from build123d import *

# Parameters (mm, degrees)
BOSS_EXTRUDE1_DEPTH      = 40
BOSS_EXTRUDE1_DEPTH_BACK = 40
SKETCH1_W                = 30
SKETCH1_H                = 40
CUT_EXTRUDE1_DEPTH       = 80
CUT_EXTRUDE1_DEPTH_BACK  = 80
SKETCH2_R                = 4.05
CUT_EXTRUDE2_START       = 15
SKETCH3_R                = 7
CUT_EXTRUDE2_DEPTH       = 6
CUT_EXTRUDE3_DEPTH       = 36
CUT_EXTRUDE3_DEPTH_BACK  = 36


with BuildPart() as part:
    # Sketch1 → Boss-Extrude1 (new, two sides: drawn at the far end of the back side and taken through both)
    with BuildSketch(Plane.XY.offset(-BOSS_EXTRUDE1_DEPTH_BACK)):
        Rectangle(SKETCH1_W, SKETCH1_H)
    extrude(amount=BOSS_EXTRUDE1_DEPTH + BOSS_EXTRUDE1_DEPTH_BACK)

    # Sketch2 → Cut-Extrude1 (cut, two sides: drawn at the far end of the back side and taken through both)
    with BuildSketch(Plane(origin=(0, 0, 0), x_dir=(0, 0, -1), z_dir=(1, 0, 0)).offset(-CUT_EXTRUDE1_DEPTH_BACK)):
        with Locations((-20, 0)):
            Circle(SKETCH2_R)
        with Locations((20, 0)):
            Circle(SKETCH2_R)
    extrude(amount=CUT_EXTRUDE1_DEPTH + CUT_EXTRUDE1_DEPTH_BACK, mode=Mode.SUBTRACT)

    # Sketch3 → Cut-Extrude2 (cut)
    with BuildSketch(Plane(origin=(0, 0, 0), x_dir=(0, 0, -1), z_dir=(1, 0, 0)).offset(CUT_EXTRUDE2_START)):
        with Locations((-20, 0)):
            Circle(SKETCH3_R)
        with Locations((20, 0)):
            Circle(SKETCH3_R)
    extrude(amount=-CUT_EXTRUDE2_DEPTH, mode=Mode.SUBTRACT)

    # Sketch4 → Cut-Extrude3 (cut, two sides: drawn at the far end of the back side and taken through both)
    with BuildSketch(Plane(origin=(0, 0, 0), x_dir=(1, 0, 0), z_dir=(0, 1, 0)).offset(-CUT_EXTRUDE3_DEPTH_BACK)):
        with BuildLine():
            Line((-0.1, -7.5), (-0.1, 7.5))
            ThreePointArc((-0.1, 7.5), (4, 11.6), (8.1, 7.5))
            Line((8.1, 7.5), (8.1, -7.5))
            ThreePointArc((8.1, -7.5), (4, -11.6), (-0.1, -7.5))
        make_face()
    extrude(amount=CUT_EXTRUDE3_DEPTH + CUT_EXTRUDE3_DEPTH_BACK, mode=Mode.SUBTRACT)


solid = part.part
Here's how the part is built. I have some questions about the finished solid (model axes, mm). A direction names the side the tool comes from. Coordinates: 2 decimals unless noted, no trailing zeros. Loops run counter-clockwise (first coordinate to the right, second up) from the corner with the lowest first, then second, coordinate; pieces in that order, holes last.
1. Imagine slicing it at A-A, the plane x = 4. Please give me the cut outline in (y, z), and give its area (3 significant figures).
2. For P1, Ø13, axis at y = 0, z = 20, coming from the +X side, with a flat end and sliding along its axis, tell me the tip position at first contact or that it passes through.
3. I need wall thicknesses on L1, parallel to Z at x = -6.5, y = 0; L2, parallel to X at y = -13.5, z = 7; L3, parallel to Y at x = -3.5, z = -20. Which ranges of each line are inside material? Lowest first, please.
4. Imagine slicing it at D-D, the plane y = 14. Please give me the cut outline in (x, z), and give its area (3 significant figures).
5. For faces 5 (the flat face through (9, -3, -23)), 6 (the cylindrical face through (-3.168, 0.178, -15.954)), 7 (the flat face through (8.1, 0, 0)), which set-ups out of +Z, -Z, +X, -X, +Y, -Y let a thin tool reach every point of the face, with its end or its side?
6. If we mould it in two halves opening along Y, with no side actions, what happens to faces 1 (the cylindrical face through (-3.168, 0.178, 24.046)), 2 (the flat face through (-4, 20, -1)), 3 (the cylindrical face through (12, 0, 27)), 4 (the flat face through (0, 0, -40))? For each: pulls with the +Y half, pulls with the -Y half, needs draft (parallel to the pull), parting line crosses it, or undercut.
7. Imagine slicing it at B-B, the plane z = 20. Please give me the cut outline in (x, y), and give its area (3 significant figures).
8. Imagine slicing it at C-C, the plane y = 0. Please give me the cut outline in (x, z), and give its area (3 significant figures).
Taken from the geometry:
1. outline: (-20, -40) - (20, -40) - (20, -11.6) - (-20, -11.6) - close; (-20, 11.6) - (20, 11.6) - (20, 40) - (-20, 40) - close; hole circle Ø8.1 at (0, -20); hole circle Ø8.1 at (0, 20)
1. area: 2,170 mm2
2. P1: stops at x = 9
3. L1: z = -40 to -24.05, -15.95 to 15.95, 24.05 to 40
3. L2: x = -15 to -0.1, 8.1 to 15
3. L3: y = -20 to -4.05, 4.05 to 20
4. outline: (-15, -40) - (15, -40) - (15, 40) - (-15, 40) - close; hole (-0.1, -7.5) arc R4.1 ccw to (8.1, -7.5) - (8.1, 7.5) arc R4.1 ccw to (-0.1, 7.5) - close
4. area: 2,220 mm2
5. face 5: +X
5. face 6: +X, -X
5. face 7: +Y, -Y
6. face 1: undercut
6. face 2: pulls with the +Y half
6. face 3: undercut
6. face 4: needs draft
7. outline: (-15, -20) - (15, -20) - (15, -7) - (9, -7) - (9, -4.05) - (-15, -4.05) - close; (-15, 4.05) - (9, 4.05) - (9, 7) - (15, 7) - (15, 20) - (-15, 20) - close
7. area: 922 mm2
8. outline: (-15, -40) - (15, -40) - (15, -27) - (9, -27) - (9, -24.05) - (-15, -24.05) - close; (-15, -15.95) - (9, -15.95) - (9, -13) - (15, -13) - (15, 13) - (9, 13) - (9, 15.95) - (-15, 15.95) - close; (-15, 24.05) - (9, 24.05) - (9, 27) - (15, 27) - (15, 40) - (-15, 40) - close; hole (-0.1, -7.5) arc R4.1 ccw to (8.1, -7.5) - (8.1, 7.5) arc R4.1 ccw to (-0.1, 7.5) - close
8. area: 1,670 mm2
